```python
from build123d import *

# Parameters (mm, degrees)
SKETCH1_R               = 6
BOSS_EXTRUDE1_DEPTH     = 6
CUT_EXTRUDE1_DEPTH      = 1
FILLET1_R               = 1
FILLET1_OF_MIRROR1_R    = 1
SKETCH3_R               = 8
SKETCH3_R_2             = 6
BOSS_EXTRUDE2_DEPTH     = 0.5
SKETCH4_R               = 8
SKETCH4_R_2             = 6
BOSS_EXTRUDE3_DEPTH     = 0.5
CUT_EXTRUDE2_DEPTH      = 50.692614274
CUT_EXTRUDE2_DEPTH_BACK = 50.692614274
SKETCH5_R               = 1.5


with BuildPart() as part:
    # Sketch1 → Boss-Extrude1 (new, symmetric)
    with BuildSketch(Plane(origin=(0, 0, 0), x_dir=(0, 0, -1), z_dir=(1, 0, 0))):
        with BuildLine():
            Line((-12.96472382, -3.473887278), (-30.667194256, -8.217249935))
            ThreePointArc((-30.667194256, -8.217249935), (-33.214466382, -10.301810854), (-33.335907835, -13.591072395))
            ThreePointArc((-33.335907835, -13.591072395), (0, -36), (33.335907835, -13.591072395))
            ThreePointArc((33.335907835, -13.591072395), (33.214466382, -10.301810854), (30.667194256, -8.217249935))
            Line((30.667194256, -8.217249935), (12.96472382, -3.473887278))
            ThreePointArc((12.96472382, -3.473887278), (10.826586639, -2.045229688), (10, 0.389816028))
            Line((10, 0.389816028), (10, 24.392304845))
            ThreePointArc((10, 24.392304845), (9.464101615, 26.392304845), (8, 27.856406461))
            ThreePointArc((8, 27.856406461), (0, 30), (-8, 27.856406461))
            ThreePointArc((-8, 27.856406461), (-9.464101615, 26.392304845), (-10, 24.392304845))
            Line((-10, 24.392304845), (-10, 0.389816028))
            ThreePointArc((-10, 0.389816028), (-10.826586639, -2.045229688), (-12.96472382, -3.473887278))
        make_face()
        Circle(SKETCH1_R, mode=Mode.SUBTRACT)
        with Locations((0, 18)):
            Circle(SKETCH1_R, mode=Mode.SUBTRACT)
    extrude(amount=BOSS_EXTRUDE1_DEPTH, both=True)

    # Sketch2 → Cut-Extrude1 (cut, symmetric)
    with BuildSketch(Plane(origin=(6, 0, 0), x_dir=(0, 0, -1), z_dir=(1, 0, 0))):
        with BuildLine():
            ThreePointArc((-12.037997029, -6.331400124), (-9.894070596, -6.35181127), (-8.068661956, -7.476409181))
            ThreePointArc((-8.068661956, -7.476409181), (0, -11), (8.068661956, -7.476409181))
            ThreePointArc((8.068661956, -7.476409181), (9.894070596, -6.35181127), (12.037997029, -6.331400124))
            Line((12.037997029, -6.331400124), (12.188266684, -6.371664756))
            Line((12.188266684, -6.371664756), (29.89073712, -11.115027414))
            ThreePointArc((29.89073712, -11.115027414), (30.527555152, -11.636167644), (30.557915515, -12.458483029))
            ThreePointArc((30.557915515, -12.458483029), (0, -33), (-30.557915515, -12.458483029))
            ThreePointArc((-30.557915515, -12.458483029), (-30.527555152, -11.636167644), (-29.89073712, -11.115027414))
            Line((-29.89073712, -11.115027414), (-12.188266684, -6.371664756))
            Line((-12.188266684, -6.371664756), (-12.037997029, -6.331400124))
        make_face()
    cut_extrude1 = extrude(amount=CUT_EXTRUDE1_DEPTH, both=True, mode=Mode.SUBTRACT)

    # Fillet1
    fillet1_edges = [part.edges().sort_by_distance(p)[0] for p in [
        (5, -11, 0),
        (5, -6.35181127, -9.894070596),
        (5, -8.723213769, -20.964367075),
        (5, -11.636167644, -30.527555152),
        (5, -33, 0),
        (5, -11.636167644, 30.527555152),
        (5, -8.723213769, 20.964367075),
        (5, -6.35181127, 9.894070596),
    ]]
    fillet(fillet1_edges, radius=FILLET1_R - 0.0001)  # a hair under: the kernel refuses the full size

    # Mirror1: Cut-Extrude1 across plane
    add(cut_extrude1.mirror(Plane(origin=(0, 0, 0), x_dir=(0, 0, 1), z_dir=(1, 0, 0))), mode=Mode.SUBTRACT)

    # Fillet1 of Mirror1
    fillet1_of_mirror1_edges = [part.edges().sort_by_distance(p)[0] for p in [
        (-5, -11, 0),
        (-5, -6.35181127, -9.894070596),
        (-5, -8.723213769, -20.964367075),
        (-5, -11.636167644, -30.527555152),
        (-5, -33, 0),
        (-5, -11.636167644, 30.527555152),
        (-5, -8.723213769, 20.964367075),
        (-5, -6.35181127, 9.894070596),
    ]]
    fillet(fillet1_of_mirror1_edges, radius=FILLET1_OF_MIRROR1_R - 0.0001)  # a hair under: the kernel refuses the full size

    # Sketch3 → Boss-Extrude2 (add, symmetric)
    with BuildSketch(Plane(origin=(6, 0, 0), x_dir=(0, 0, -1), z_dir=(1, 0, 0))):
        with Locations(Location((0, 0, 0), (0, 0, 180))):
            Circle(SKETCH3_R)
        Circle(SKETCH3_R_2, mode=Mode.SUBTRACT)
    extrude(amount=BOSS_EXTRUDE2_DEPTH, both=True)

    # Sketch4 → Boss-Extrude3 (add, symmetric)
    with BuildSketch(Plane.ZY.offset(6)):
        with Locations((0, 18)):
            Circle(SKETCH4_R)
        with Locations((0, 18)):
            Circle(SKETCH4_R_2, mode=Mode.SUBTRACT)
    extrude(amount=BOSS_EXTRUDE3_DEPTH, both=True)

    # Sketch5 → Cut-Extrude2 (cut, two sides: drawn at the far end of the back side and taken through both)
    with BuildSketch(Plane.XY.offset(-CUT_EXTRUDE2_DEPTH_BACK)):
        with Locations((0, 18)):
            Circle(SKETCH5_R)
        Circle(SKETCH5_R)
    extrude(amount=CUT_EXTRUDE2_DEPTH + CUT_EXTRUDE2_DEPTH_BACK, mode=Mode.SUBTRACT)


solid = part.part
```
Build history of the part. All positions in model axes, mm. A direction names the side the tool comes from. Round coordinates to 2 decimals unless told otherwise and drop trailing zeros. Write each loop counter-clockwise with the first axis right and the second up, starting at its lowest first coordinate (ties: lowest second). Pieces come first, ordered by that corner, then holes.
1) Drill centre lines: probe 1 along Y at (x, z) = (-1.25, 0); probe 2 along X at (y, z) = (18, 7.4); probe 3 along Y at (x, z) = (0, 8.15). Where is each one in solid material? Low to high.
2) 3-axis set-ups, long thin cutter, end or side, ignore diameter. For faces 1 (the flat face through (0, 12, -10)), 2 (the cylindrical face through (-6.25, 10.19, -1.73)), 3 (the cylindrical face through (-0.325, -1.464, -8.175)): which of +Z, -Z, +X, -X, +Y, -Y reach the whole face in a straight line?
3) Band-saw the part on A-A, the plane x = 0. List the corners of the cut face in (y, z), and give its area (3 significant figures).
4) Band-saw the part on B-B, the plane z = 0. Give the number of separate pieces and of enclosed holes in the cut face, and give its area (3 significant figures).
5) Mould opens along Y. For faces 4 (the cylindrical face through (-0.195, 19.487, -7.934)), 5 (the cylindrical face through (0.084, 26.367, -9.479)), 6 (the cylindrical face through (0.084, -10.259, 33.193)) say: +Y half, -Y half, draft (parallel to the pull), parting line (faces both ways), or undercut.
6) Pin check, flat tips, straight feed: pin 1 (7 mm diameter, centred on y = 18, z = 0, fed in from +X); pin 2 (1.5 mm diameter, centred on x = 3, z = 12, fed in from +Y); pin 3 (6 mm diameter, centred on x = 4, z = -15, fed in from +Y); pin 4 (5 mm diameter, centred on x = 0, y = 18, fed in from -Z). Stop position of each tip, or through.
Ans:
1. probe 1: y = -36 to -6, 6 to 12, 24 to 30
1. probe 2: x = -6.5 to -1.5, 1.5 to 6
1. probe 3: y = -35.07 to -1.5, 1.5 to 16.5, 19.5 to 27.77
2. face 1: -Z, +X, -X, +Y
2. face 2: -X
2. face 3: +Z, -Z
3. outline: (-13.59, -33.34) arc R4 ccw to (-8.22, -30.67) - (-3.47, -12.96) arc R4 cw to (-1.5, -10.47) - (-1.5, -5.81) arc R6 cw to (-1.5, 5.81) - (-1.5, 10.47) arc R4 cw to (-3.47, 12.96) - (-8.22, 30.67) arc R4 ccw to (-13.59, 33.34) arc R36 ccw to start; (1.5, -10) - (16.5, -10) - (16.5, -5.81) arc R6 cw to (16.5, 5.81) - (16.5, 10) - (1.5, 10) - (1.5, 5.81) arc R6 cw to (1.5, -5.81) - close; (19.5, -10) - (24.39, -10) arc R4 ccw to (27.86, -8) arc R16 ccw to (27.86, 8) arc R4 ccw to (24.39, 10) - (19.5, 10) - (19.5, 5.81) arc R6 cw to (19.5, -5.81) - close
3. area: 2,020 mm2
4. separate pieces: 3
4. enclosed holes: 0
4. area: 465 mm2
5. face 4: undercut
5. face 5: +Y half
5. face 6: parting line
6. pin 1: passes through
6. pin 2: stops at y = -2.51
6. pin 3: stops at y = -3.07
6. pin 4: stops at z = -10
